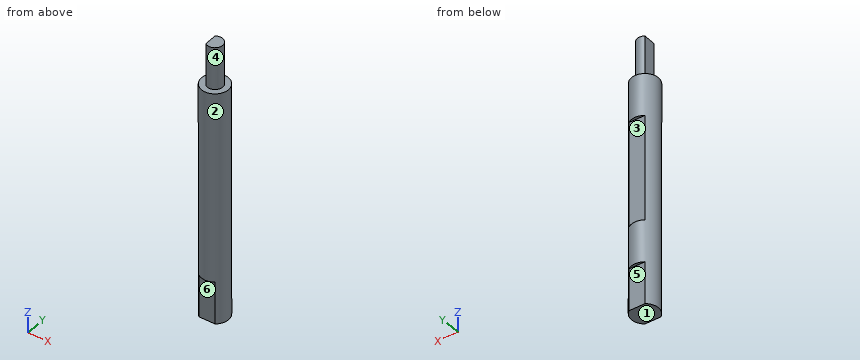
```python
from build123d import *

# Parameters (mm, degrees)
SKETCH1_R           = 3.175
BOSS_EXTRUDE1_DEPTH = 65
CUT_EXTRUDE1_DEPTH  = 10
CUT_EXTRUDE2_DEPTH  = 25
CUT_EXTRUDE3_START  = -10
SKETCH4_R           = 3.175
CUT_EXTRUDE3_DEPTH  = 10


with BuildPart() as part:
    # Sketch1 → Boss-Extrude1 (new body)
    with BuildSketch(Plane.XY):
        Circle(SKETCH1_R)
    extrude(amount=BOSS_EXTRUDE1_DEPTH)

    # Sketch2 → Cut-Extrude1 (cut)
    with BuildSketch(Plane(origin=(0, 0, 0), x_dir=(-1, 0, 0), z_dir=(0, 0, -1))):
        with BuildLine():
            Line((-1.891593244, 2.55), (1.891593244, 2.55))
            ThreePointArc((1.891593244, 2.55), (0, 3.175), (-1.891593244, 2.55))
        make_face()
        with BuildLine():
            Line((-1.891593244, -2.55), (1.891593244, -2.55))
            ThreePointArc((1.891593244, -2.55), (0, -3.175), (-1.891593244, -2.55))
        make_face()
    extrude(amount=-CUT_EXTRUDE1_DEPTH, mode=Mode.SUBTRACT)

    # Sketch3 → Cut-Extrude2 (cut)
    with BuildSketch(Plane(origin=(0, 0, 20), x_dir=(-1, 0, 0), z_dir=(0, 0, -1))):
        with BuildLine():
            Line((-1.891593244, 2.55), (1.891593244, 2.55))
            ThreePointArc((1.891593244, 2.55), (0, 3.175), (-1.891593244, 2.55))
        make_face()
    extrude(amount=-CUT_EXTRUDE2_DEPTH, mode=Mode.SUBTRACT)

    # Sketch4 → Cut-Extrude3 (cut)
    with BuildSketch(Plane.XY.offset(65).offset(CUT_EXTRUDE3_START)):
        with Locations(Location((0, 0, 0), (0, 0, 126.568071017))):
            Circle(SKETCH4_R)
        with BuildLine():
            Line((-1.073, -1.478715659), (-1.073, 1.478715659))
            ThreePointArc((-1.073, 1.478715659), (1.827, 0), (-1.073, -1.478715659))
        make_face(mode=Mode.SUBTRACT)
    extrude(amount=CUT_EXTRUDE3_DEPTH, mode=Mode.SUBTRACT)


solid = part.part
```
Can you work these out from the model? Positions are in its coordinate system, mm. Face numbers are marked on the shaded views. A direction names the side the tool comes from. Round coordinates to 2 decimals unless told otherwise and drop trailing zeros. Order: outer loops, then holes, each group sorted by start corner. A loop starts at its lowest first (then second) coordinate and runs counter-clockwise, first axis right, second up. Notation, with made-up numbers: (57, 77.5) -> (86, 77.5) arc R14 cw to (86, 90.5) -> close; hole circle Ø2 at (68.5, 28.5). An arc over 180 degrees is marked (long way). Return JSON: item names as keys, results as strings. Group by question number.
1. Which directions (+Z, -Z, +X, -X, +Y, -Y) give clear straight access to the entire face, cutting with the end or side of a thin tool? Please do the marked faces 4, 5 and 6.
2. If we section it at B-B, the plane y = 0: Write out the boundary of the cut face in (x, z) (3 decimals).
3. If we section it at D-D, the plane z = 48: Write out the boundary of the cut face in (x, y) (3 decimals).
4. If we section it at A-A, the plane x = 0: Write out the boundary of the cut face in (y, z) (3 decimals), then the cut area to 3 significant figures.
5. We'd pull the mould along Z, two halves only. Please class the marked faces 1, 2 and 3: released by +Z, released by -Z, zero draft, split by the parting line, or undercut.
6. Will these pins go through, and if not, where does the flat tip stop? pin 1 (1.9 mm diameter, centred on x = 0, z = 6, fed in from +Y); pin 2 (1.1 mm diameter, centred on x = -0.5, z = 7.5, fed in from -Y); pin 3 (2.5 mm diameter, centred on y = 0.5, z = 58, fed in from -X).
7. I need wall thicknesses on line 1 (Z direction, x = 2, y = -1); line 2 (X direction, y = 0.25, z = 35); line 3 (Z direction, x = 0.25, y = -3). Which ranges of each line are inside material? Lowest first, please. Write a range as [from, to].
8. If we section it at C-C, the plane z = 30: Write out the boundary of the cut face in (x, y) (3 decimals), then the cut area to 3 significant figures.
Output values:
{
 "1": {"face 4": "+Z", "face 5": "-Z, +X, -X, +Y", "face 6": "-Z, +X, -X, -Y"},
 "2": {"outline": "(-3.175, 0) -> (3.175, 0) -> (3.175, 55) -> (1.827, 55) -> (1.827, 65) -> (-1.073, 65) -> (-1.073, 55) -> (-3.175, 55) -> close"},
 "3": {"outline": "circle Ø6.35 at (0, 0)"},
 "4": {"outline": "(-3.175, 10) -> (-2.55, 10) -> (-2.55, 0) -> (2.55, 0) -> (2.55, 10) -> (3.175, 10) -> (3.175, 20) -> (2.55, 20) -> (2.55, 45) -> (3.175, 45) -> (3.175, 55) -> (1.827, 55) -> (1.827, 65) -> (-1.827, 65) -> (-1.827, 55) -> (-3.175, 55) -> close", "area": "358 mm²"},
 "5": {"face 1": "released by -Z", "face 2": "zero draft", "face 3": "undercut"},
 "6": {"pin 1": "y = 2.55", "pin 2": "y = -2.55", "pin 3": "x = -1.07"},
 "7": {"line 1": "[0, 55]", "line 2": "[-3.17, 3.17]", "line 3": "[10, 55]"},
 "8": {"outline": "(-1.892, 2.55) arc R3.175 ccw (long way) to (1.892, 2.55) -> close", "area": "30.1 mm²"}
}
